The model under review builds one solid part; all positions refer to its coordinate system, in mm. Face numbers are marked on the shaded views. A direction names the side the tool comes from. Coordinates: 2 decimals unless noted, no trailing zeros. Write each loop counter-clockwise with the first axis right and the second up, starting at its lowest first coordinate (ties: lowest second). Pieces come first, ordered by that corner, then holes. Notation, with made-up numbers: M 43.5,-28.5 L 91.5,-28.5 A26 cw 91.5,-4.5 Z; hole C 44,68 d6. An arc over 180 degrees is marked long. Answer as a JSON object with one key per item and string values.
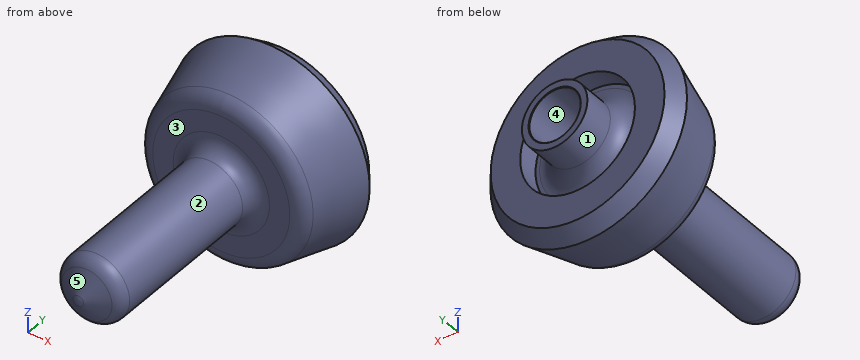
```python
from build123d import *

# Parameters (mm, degrees)
FILLET1_R                       = 1
F_2_5MM_DOWEL_HOLE1_D           = 2.5
F_2_5MM_DOWEL_HOLE1_DEPTH       = 5.5
F_2_5MM_DOWEL_HOLE1_CSINK_D     = 2.55
F_2_5MM_DOWEL_HOLE1_CSINK_ANGLE = 90
F_2_5MM_DOWEL_HOLE1_TIP         = 0.751075774


with BuildPart() as part:
    # Sketch1 → Revolve1 (revolve)
    with BuildSketch(Plane.XY, mode=Mode.PRIVATE) as revolve1_sk:
        with BuildLine():
            Line((1.6, 15), (1.6, 12.5))
            Line((1.6, 12.5), (2.8, 12.5))
            Line((2.8, 12.5), (2.8, 13.5))
            Line((2.8, 13.5), (4.244114284, 13.5))
            Line((4.244114284, 13.5), (4.8, 12.77555563))
            Line((4.8, 12.77555563), (4.071266643, 10.055885716))
            ThreePointArc((4.071266643, 10.055885716), (3.803393345, 9.654984995), (3.346822273, 9.5))
            Line((3.346822273, 9.5), (2.35, 9.5))
            ThreePointArc((2.35, 9.5), (1.819669914, 9.280330086), (1.6, 8.75))
            Line((1.6, 8.75), (1.6, 1.356773133))
            ThreePointArc((1.6, 1.356773133), (1.499519053, 0.981773133), (1.225, 0.70725408))
            Line((1.225, 0.70725408), (0.258564065, 0.149282032))
            ThreePointArc((0.258564065, 0.149282032), (0.133842609, 0.097620714), (0, 0.08))
            Line((0, 0.08), (0, 15))
            Line((0, 15), (1.6, 15))
        make_face()
    revolve(revolve1_sk.sketch.rotate(Axis((0, 17.798555487, 0), (0, -1, 0)), 180), axis=Axis((0, 17.798555487, 0), (0, -1, 0)))

    # Fillet1
    fillet1_edges = [part.edges().sort_by_distance(p)[0] for p in [
        (1.6, 12.5, 0),
    ]]
    fillet(fillet1_edges, radius=FILLET1_R)

    # Ø2.5mm Dowel Hole1
    with Locations(Plane(origin=(0, 15, 0), x_dir=(1, 0, 0), z_dir=(0, 1, 0))):
        with Locations((0, 0)):
            CounterSinkHole(F_2_5MM_DOWEL_HOLE1_D / 2, F_2_5MM_DOWEL_HOLE1_CSINK_D / 2, depth=F_2_5MM_DOWEL_HOLE1_DEPTH, counter_sink_angle=F_2_5MM_DOWEL_HOLE1_CSINK_ANGLE)
            with Locations((0, 0, -(F_2_5MM_DOWEL_HOLE1_DEPTH + F_2_5MM_DOWEL_HOLE1_TIP / 2))):  # 118° drill point
                Cone(0, F_2_5MM_DOWEL_HOLE1_D / 2, F_2_5MM_DOWEL_HOLE1_TIP, mode=Mode.SUBTRACT)


solid = part.part
```
(1) Wall thickness on line 1 along Z through (x, y) = (0, 13.05); line 2 along Z through (x, y) = (0, 13.1); line 3 along Y through (x, z) = (-2.5, -0.5): over which ranges is each line inside the solid? List them lowest first. Write a range as from..to.
Results list:
{"line 1": "-4.59..-2.8, -1.71..-1.25, 1.25..1.71, 2.8..4.59", "line 2": "-4.55..-2.8, -1.68..-1.25, 1.25..1.68, 2.8..4.55", "line 3": "9.5..12.5"}
(2) Add section A-A on y = 1.75. Give the boundary of the cut face in (x, z), and give its area (3 significant figures).
Results list:
{"outline": "C 0,0 d3.2", "area": "8.04 mm²"}
(3) Draft analysis for pull direction X (two halves, no side actions). For the marked faces 3, 4 and 5, state which applies: released by +X, released by -X, zero draft, split by the parting line, or undercut.
Results list:
{"face 3": "zero draft", "face 4": "undercut", "face 5": "split by the parting line"}
(4) For the marked faces 1 and 2, list the 3-axis set-ups (+Z, -Z, +X, -X, +Y, -Y) from which the entire face can be reached by the end or side of a thin tool; tool diameter is ignored.
Results list:
{"face 1": "+Y", "face 2": "-Y"}
(5) For pin 1 Ø3 at (x, y) = (2.5, 2) entering from +Z; pin 2 Ø5 at (y, z) = (5.5, -1) entering from -X; pin 3 Ø1.5 at (x, y) = (-0.5, 12) entering from -Z, all flat-tipped, find the tip position at first contact; note any pin that passes through.
Results list:
{"pin 1": "z = 1.25", "pin 2": "x = -1.6", "pin 3": "z = -4.78"}
